The model under review builds one solid part; all positions refer to its coordinate system, in mm. A direction names the side the tool comes from. Coordinates: 2 decimals unless noted, no trailing zeros. Write each loop counter-clockwise with the first axis right and the second up, starting at its lowest first coordinate (ties: lowest second). Pieces come first, ordered by that corner, then holes.
```python
from build123d import *

# Parameters (mm, degrees)
F0_W     = 33
F0_H     = 33
F0_R     = 9.5
F1_DEPTH = 10
F2_R     = 4
F4_DEPTH = 500


with BuildPart() as f1:
    # F0 (on Front) → F1 (new body)
    with BuildSketch(Plane.XZ):
        Rectangle(F0_W, F0_H)
        Circle(F0_R, mode=Mode.SUBTRACT)
    extrude(amount=F1_DEPTH)

    # F2
    f2_edges = [f1.edges().sort_by_distance(p)[0] for p in [
        (0, -10, 16.5),
        (16.5, -10, 0),
        (-16.5, -10, 0),
        (0, -10, -16.5),
        (-16.5, -5, 16.5),
        (16.5, -5, 16.5),
        (16.5, -5, -16.5),
        (-16.5, -5, -16.5),
    ]]
    fillet(f2_edges, radius=F2_R)

    # F3 (on face) → F4 (cut)
    with BuildSketch(Plane.XY.offset(16.5)):
        with BuildLine():
            Line((-12.5, 0), (-12.5, -0.76783))
            ThreePointArc((-12.5, -0.76783), (0, -1.28957), (12.5, -0.76783))
            Line((12.5, -0.76783), (12.5, 0))
            Line((12.5, 0), (-12.5, 0))
        make_face()
        with BuildLine():
            ThreePointArc((12.5, -0.76783), (110.397011, 47.15995), (150, 148.71043))
            ThreePointArc((150, 148.71043), (-101.55048, 259.10744), (-12.5, -0.76783))
            Line((-12.5, -0.76783), (-12.5, 0))
            Line((-12.5, 0), (12.5, 0))
            Line((12.5, 0), (12.5, -0.76783))
        make_face()
    extrude(amount=-F4_DEPTH, mode=Mode.SUBTRACT)


solid = f1.part
```
Item 1: Mouldability with a two-part tool opening along X and no side actions: class faces 1 (the face through (15.297, -3.229, 15.359)), 2 (the face through (-14.529, -0.584, 0.231)), 3 (the face through (-0.18, -1.29, -10.77)), 4 (the face through (-15.359, -3.229, -15.297)) as pulls with the +X half, pulls with the -X half, needs draft (parallel to the pull), parting line crosses it, or undercut.
Solved:
face 1: pulls with the +X half
face 2: undercut
face 3: undercut
face 4: pulls with the -X half
Item 2: Take a section at D-D, the plane x = -5.5. Write out the cut boundary in (y, z).
Solved:
outline: (-10, -12.5) arc R4 ccw to (-6, -16.5) - (-1.19, -16.5) - (-1.19, -7.75) - (-10, -7.75) - close; (-10, 7.75) - (-1.19, 7.75) - (-1.19, 16.5) - (-6, 16.5) arc R4 ccw to (-10, 12.5) - close
Item 3: Take a section at B-B, the plane x = 0. Write out the cut boundary in (y, z), plus the area to 3 significant figures.
Solved:
outline: (-10, -12.5) arc R4 ccw to (-6, -16.5) - (-1.29, -16.5) - (-1.29, -9.5) - (-10, -9.5) - close; (-10, 9.5) - (-1.29, 9.5) - (-1.29, 16.5) - (-6, 16.5) arc R4 ccw to (-10, 12.5) - close
area: 115 mm2
Item 4: To check wall thickness, follow line 1 along X through (y, z) = (-1.75, 0); line 2 along X through (y, z) = (-7.25, -7). State the ranges of each line that lie inside material, in increasing order.
Solved:
line 1: x = -16.5 to -9.5, 9.5 to 16.5
line 2: x = -16.3 to -6.42, 6.42 to 16.3
Item 5: Take a section at A-A, the plane z = 0. Write out the cut boundary in (x, y).
Solved:
outline: (-16.5, -6) arc R4 ccw to (-12.5, -10) - (-9.5, -10) - (-9.5, -0.99) arc R150 cw to (-12.5, -0.77) arc R150 cw to (-16.5, -0.38) - close; (9.5, -10) - (12.5, -10) arc R4 ccw to (16.5, -6) - (16.5, -0.38) arc R150 cw to (12.5, -0.77) arc R150 cw to (9.5, -0.99) - close
Item 6: Machinability: for faces 5 (the face through (-15.359, -3.229, 15.297)), 6 (the face through (14.47, -0.59, 0.23)), which of the approach directions +Z, -Z, +X, -X, +Y, -Y give a long, thin tool a straight path to every point of the face, cutting with its end or side? Answer none if there is none.
Solved:
face 5: +Z, -X, +Y, -Y
face 6: +Z, -Z, +Y
Item 7: Take a section at C-C, the plane y = -4. Write out the cut boundary in (x, z), plus the area to 3 significant figures.
Solved:
outline: (-16.5, -12.5) arc R4 ccw to (-12.5, -16.5) - (12.5, -16.5) arc R4 ccw to (16.5, -12.5) - (16.5, 12.5) arc R4 ccw to (12.5, 16.5) - (-12.5, 16.5) arc R4 ccw to (-16.5, 12.5) - close; hole circle Ø19 at (0, 0)
area: 792 mm2
Item 8: For pin 1 (6 mm diameter, centred on x = 0.5, z = 9, fed in from +Y); pin 2 (3 mm diameter, centred on x = -9.5, y = -8, fed in from +Z), all flat-tipped, find the tip position at first contact; note any pin that passes through.
Solved:
pin 1: stops at y = -1.25
pin 2: stops at z = 16.47
